Check sheet for the modelled part. Datum: model origin and axes. Units: mm. Face numbers are marked on the shaded views. A direction names the side the tool comes from. Coordinates: 2 decimals unless noted, no trailing zeros. Loops run counter-clockwise (first coordinate to the right, second up) from the corner with the lowest first, then second, coordinate; pieces in that order, holes last. Notation, with made-up numbers: (43.5, 21.5) -> (100.5, 21.5) arc R25 ccw to (100.5, 51.5) -> close; hole circle Ø2 at (85.25, 10). An arc over 180 degrees is marked (long way). Use CSV: the item, a comma, the result in double quotes. Start each with the question number.
1. Release check for a two-part mould opening along X. For the marked faces 1, 2 and 3 record: pulls with the +X half, pulls with the -X half, needs draft (parallel to the pull), parting line crosses it, or undercut.
2. Sectioned sample at D-D, the plane x = 0. Record the cut outline in (y, z).
3. Sectioned sample at B-B, the plane z = 152.5. Record the cut outline in (x, y), and give its area (3 significant figures).
4. Set-up check for the marked faces 4 and 5: record each of +Z, -Z, +X, -X, +Y, -Y from which the full face is reachable in a straight line by a thin tool's end or side.
5. Sectioned sample at C-C, the plane y = -109. Record the cut outline in (x, z), and give its area (3 significant figures).
6. Gauge pin test, flat ends, axial feed: pin 1 (1.6 mm diameter, centred on x = -126.5, z = 24, fed in from -Y); pin 2 (1 mm diameter, centred on x = 18, z = 108.5, fed in from -Y); pin 3 (22 mm diameter, centred on x = 131, y = -113, fed in from -Z). Record the tip position at first contact, or that the pin passes through.
7. Sectioned sample at A-A, the plane y = -36. Record the cut outline in (x, z).
8. Thickness scan on L1, parallel to X at y = -97.5, z = 138; L2, parallel to X at y = 23.5, z = 36; L3, parallel to Y at x = 76, z = 68. Record the ranges inside material, lowest first.
```python
from build123d import *

# Parameters (mm, degrees)
BASE_FLANGE1_DEPTH  = 185
EXTRUDE1_DEPTH      = 353.615938381
EXTRUDE1_DEPTH_BACK = 353.615938381
SKETCH10_W          = 45
SKETCH10_H          = 40


# Sheet-metal steps are written as plain solids
with BuildPart() as part:
    # Sketch1 → Base-Flange1 (new body)
    with BuildSketch(Plane.XY):
        with BuildLine():
            Line((145, -125), (129, -125))
            ThreePointArc((129, -125), (126.171572875, -123.828427125), (125, -121))
            Line((125, -121), (125, 0))
            ThreePointArc((125, 0), (0, 125), (-125, 0))
            Line((-125, 0), (-125, -121))
            ThreePointArc((-125, -121), (-126.171572875, -123.828427125), (-129, -125))
            Line((-129, -125), (-145, -125))
            Line((-145, -125), (-145, -123))
            Line((-145, -123), (-129, -123))
            ThreePointArc((-129, -123), (-127.585786438, -122.414213562), (-127, -121))
            Line((-127, -121), (-127, 0))
            ThreePointArc((-127, 0), (0, 127), (127, 0))
            Line((127, 0), (127, -121))
            ThreePointArc((127, -121), (127.585786438, -122.414213562), (129, -123))
            Line((129, -123), (145, -123))
            Line((145, -123), (145, -125))
        make_face()
    extrude(amount=BASE_FLANGE1_DEPTH)

    # Sketch10 → Extrude1 (cut, two sides: drawn at the far end of the back side and taken through both)
    with BuildSketch(Plane(origin=(127, 0, 0), x_dir=(0, 0, -1), z_dir=(1, 0, 0)).offset(-EXTRUDE1_DEPTH_BACK)):
        with Locations((-22.5, -105)):
            Rectangle(SKETCH10_W, SKETCH10_H)
    extrude(amount=EXTRUDE1_DEPTH + EXTRUDE1_DEPTH_BACK, mode=Mode.SUBTRACT)


solid = part.part
```
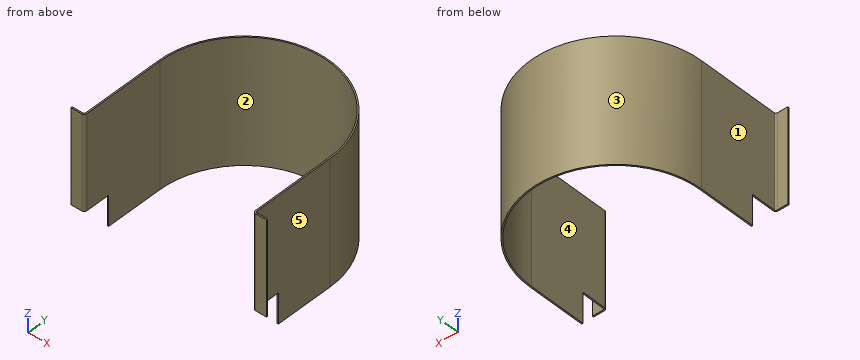
Completed:
1,face 1,"pulls with the -X half"
1,face 2,"undercut"
1,face 3,"parting line crosses it"
2,outline,"(125, 0) -> (127, 0) -> (127, 185) -> (125, 185) -> close"
3,outline,"(-145, -125) -> (-129, -125) arc R4 ccw to (-125, -121) -> (-125, 0) arc R125 cw to (125, 0) -> (125, -121) arc R4 ccw to (129, -125) -> (145, -125) -> (145, -123) -> (129, -123) arc R2 cw to (127, -121) -> (127, 0) arc R127 ccw to (-127, 0) -> (-127, -121) arc R2 cw to (-129, -123) -> (-145, -123) -> close"
3,area,"1,360 mm²"
4,face 4,"+Z, -Z, -Y"
4,face 5,"+Z, -Z, +X, +Y"
5,outline,"(-127, 45) -> (-125, 45) -> (-125, 185) -> (-127, 185) -> close; (125, 45) -> (127, 45) -> (127, 185) -> (125, 185) -> close"
5,area,"560 mm²"
6,pin 1,"y = -85"
6,pin 2,"y = 123.62"
6,pin 3,"z = 45"
7,outline,"(-127, 0) -> (-125, 0) -> (-125, 185) -> (-127, 185) -> close; (125, 0) -> (127, 0) -> (127, 185) -> (125, 185) -> close"
8,L1,"-127 to -125, 125 to 127"
8,L2,"-124.81 to -122.77, 122.77 to 124.81"
8,L3,"99.24 to 101.75"
